Study the drawing (mm; zero at the part's minimum x, y, z) and answer. A direction names the side the tool comes from. Coordinates: 2 decimals unless noted, no trailing zeros. Write each loop counter-clockwise with the first axis right and the second up, starting at its lowest first coordinate (ties: lowest second). Pieces come first, ordered by that corner, then holes. Notation, with made-up numbers: (13.25, 56) - (29.25, 56) arc R20 ccw to (29.25, 89) - close; hole circle Ø10 at (2.5, 51.25). An arc over 180 degrees is marked (long way). One line per item, written item: value.
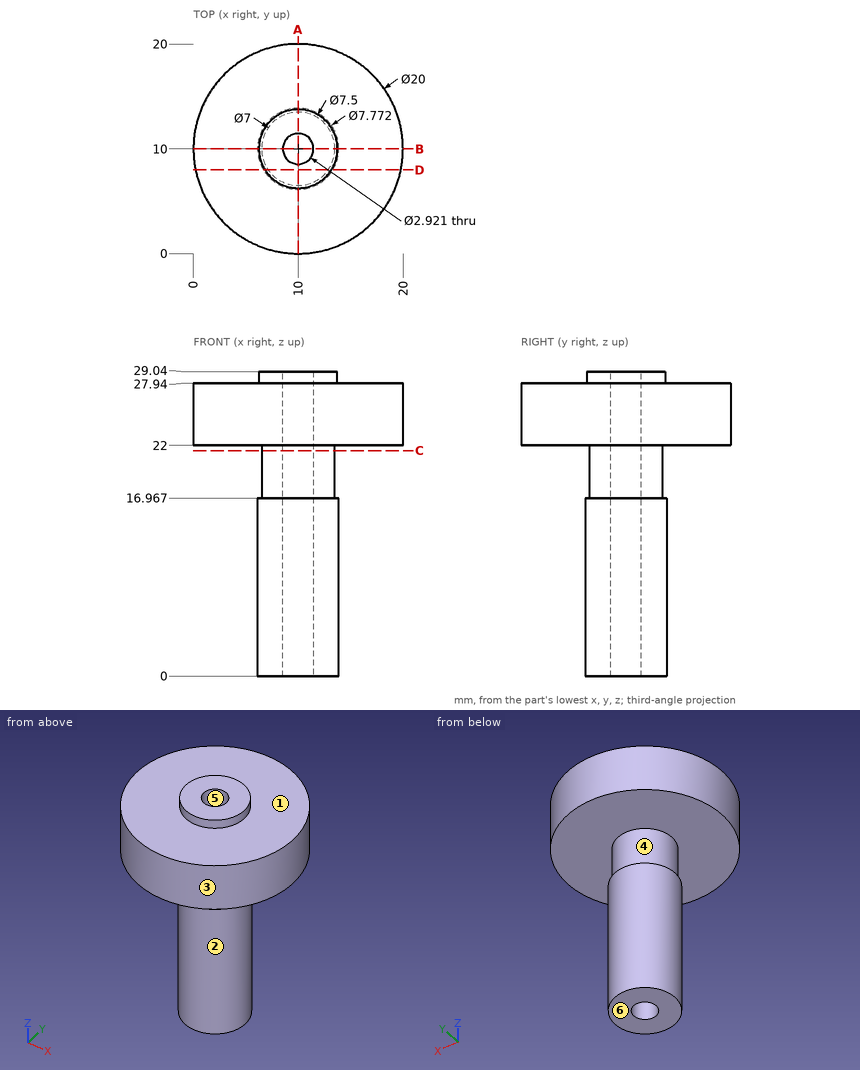
Item 1: Section C-C, the plane z = 21.5 is taken. Determine the outline of the cut face in (x, y), then the cut area to 3 significant figures.
Evaluation:
outline: circle Ø7 at (10, 10); hole circle Ø2.92 at (10, 10)
area: 31.8 mm2
Item 2: Section A-A, the plane x = 10 is taken. Determine the outline of the cut face in (y, z), then the cut area to 3 significant figures.
Evaluation:
outline: (0, 22) - (6.5, 22) - (6.5, 16.97) - (6.11, 16.97) - (6.11, 0) - (8.54, 0) - (8.54, 29.04) - (6.25, 29.04) - (6.25, 27.94) - (0, 27.94) - close; (11.46, 0) - (13.89, 0) - (13.89, 16.97) - (13.5, 16.97) - (13.5, 22) - (20, 22) - (20, 27.94) - (13.75, 27.94) - (13.75, 29.04) - (11.46, 29.04) - close
area: 209 mm2
Item 3: Section D-D, the plane y = 8 is taken. Determine the outline of the cut face in (x, z).
Evaluation:
outline: (0.2, 22) - (7.13, 22) - (7.13, 16.97) - (6.67, 16.97) - (6.67, 0) - (13.33, 0) - (13.33, 16.97) - (12.87, 16.97) - (12.87, 22) - (19.8, 22) - (19.8, 27.94) - (13.17, 27.94) - (13.17, 29.04) - (6.83, 29.04) - (6.83, 27.94) - (0.2, 27.94) - close
Item 4: Consider probe 1 along Y at (x, z) = (10, 7.25); probe 2 along Y at (x, z) = (10, 17.5); probe 3 along Z at (x, y) = (16.25, 10.25). Determine where each line is inside the solid, lowest interval first.
Evaluation:
probe 1: y = 6.11 to 8.54, 11.46 to 13.89
probe 2: y = 6.5 to 8.54, 11.46 to 13.5
probe 3: z = 22 to 27.94
Item 5: Given pin 1 (6 mm diameter, centred on y = 7, z = 20.5, fed in from -X); pin 2 (1.5 mm diameter, centred on x = 13.5, y = 2, fed in from +Z); pin 3 (8 mm diameter, centred on y = 14, z = 13, fed in from +X), each flat-ended and moving along its own axis, determine where each tip first touches the part or whether it passes through.
Evaluation:
pin 1: stops at x = 0.01
pin 2: stops at z = 27.94
pin 3: stops at x = 13.89
Item 6: Determine the mould class of the marked faces 4, 5 and 6 for opening direction Y: +Y half, -Y half, draft (parallel to the pull), parting line (faces both ways), or undercut.
Evaluation:
face 4: parting line
face 5: undercut
face 6: draft
Item 7: Which of the six approach directions +Z, -Z, +X, -X, +Y, -Y give full straight-line access (tool end or side, diameter ignored) to the marked faces 1, 2 and 3?
Evaluation:
face 1: +Z
face 2: -Z
face 3: +Z, -Z
